from build123d import *

# Parameters (mm, degrees)
F0_R      = 19.7846022737
F1_DEPTH  = 2.794
F1_FACE_R = 19.7846022737
F2_DEPTH  = 6.43804
F2_TAPER  = 45
F2_FACE_R = 13.3465622737
F3_DEPTH  = 12.08628
F3_TAPER  = 3
F4_R      = 10.241679593
F5_DEPTH  = 2.95594
F6_R      = 0.762
F7_R      = 5.08
F8_T      = -2.54
F9_R      = 7.1796509853
F10_DEPTH = 15.93384
F10_TAPER = 3
F11_R     = 4.6826437898
F12_DEPTH = 8.40654


with BuildPart() as f1:
    # F0 (on Top) → F1 (new body)
    with BuildSketch(Plane.XY):
        Circle(F0_R)
    extrude(amount=F1_DEPTH)

    # F1_face (on face) → F2 (join)
    with BuildSketch(Plane.XY.offset(2.794)):
        Circle(F1_FACE_R)
    extrude(amount=F2_DEPTH, taper=F2_TAPER)

    # F2_face (on face) → F3 (join)
    with BuildSketch(Plane.XY.offset(9.23204)):
        Circle(F2_FACE_R)
    extrude(amount=F3_DEPTH, taper=F3_TAPER)

    # F4 (on face) → F5 (cut, symmetric)
    with BuildSketch(Plane.XY.offset(21.31832)):
        Circle(F4_R)
    extrude(amount=F5_DEPTH, both=True, mode=Mode.SUBTRACT)

    # F6
    f6_edges = [f1.edges().sort_by_distance(p)[0] for p in [
        (-12.713147, 0, 21.31832),
        (-10.24168, 0, 21.31832),
    ]]
    fillet(f6_edges, radius=F6_R)

    # F7
    f7_edges = [f1.edges().sort_by_distance(p)[0] for p in [
        (-10.24168, 0, 18.36238),
    ]]
    fillet(f7_edges, radius=F7_R)

    # F8
    f8_openings = [f1.faces().sort_by_distance(p)[0] for p in [
        (0, 0, 0),
    ]]
    offset(amount=F8_T, openings=f8_openings, kind=Kind.INTERSECTION)

    # F9 (on face) → F10 (join)
    with BuildSketch(Plane(origin=(0, 0, 15.82238), x_dir=(1, 0, 0), z_dir=(0, 0, -1))):
        Circle(F9_R)
    extrude(amount=F10_DEPTH, taper=F10_TAPER)

    # F11 (on face) → F12 (cut, symmetric)
    with BuildSketch(Plane(origin=(0, 0, -0.11146), x_dir=(1, 0, 0), z_dir=(0, 0, -1))):
        Circle(F11_R)
    extrude(amount=F12_DEPTH, both=True, mode=Mode.SUBTRACT)


solid = f1.part
Work out the finished part from the listing and answer in its coordinate system (mm). A direction names the side the tool comes from. Coordinates: 2 decimals unless noted, no trailing zeros. Order: outer loops, then holes, each group sorted by start corner. A loop starts at its lowest first (then second) coordinate and runs counter-clockwise, first axis right, second up. Notation, with made-up numbers: (36, 51) - (54, 51) arc R20 cw to (54, 66) - close; hole circle Ø4 at (-26.5, 26.5). An arc over 180 degrees is marked (long way). Put each result on its own line as item: value. Start each with the question number.
1) Flat-ended cylindrical pins translate along their axes: pin 1 (4 mm diameter, centred on x = -4.5, y = 7.5, fed in from +Z); pin 2 (4 mm diameter, centred on y = 14, z = 14.5, fed in from -X); pin 3 (1 mm diameter, centred on x = -6.5, z = 11, fed in from +Y); pin 4 (20.5 mm diameter, centred on x = 0, y = 0, fed in from -Z). Find the tip coordinate at first contact, or state that the pin passes through.
2) Find section B-B (z = 15). Give the vertices of the cut face in (x, y), plus the area to 3 significant figures.
3) Find the intervals of material crossed by line 1 (Y direction, x = 0, z = 1.3); line 2 (Y direction, x = 0, z = 2.5); line 3 (Y direction, x = -4, z = 12.75), in increasing order. Write a range as from..to.
4) Find section A-A (z = 6.5). Give the vertices of the cut face in (x, y).
5) Find section C-C (z = 11.5). Give the vertices of the cut face in (x, y), plus the area to 3 significant figures.
6) For faces 1 (the cylindrical face through (-3.716, 2.849, 4.033)), 2 (the conical face through (-2.961, -13.334, 8.919)), determine the directions among +Z, -Z, +X, -X, +Y, -Y from which every point of the face is accessible in a straight line to the end or side of a thin tool.
7) For a pull along X with two mould halves and no side action, classify faces 3 (the conical face through (5.989, -11.514, 16.256)), 4 (the flat face through (0, 0, 8.295)), 5 (the flat face through (5, -10, 21.318)), 6 (the flat face through (0, 0, 18.362)) as released by +X, released by -X, zero draft, split by the parting line, or undercut.
Results list:
1. pin 1: stops at z = 21.27
1. pin 2: stops at x = -5.19
1. pin 3: stops at y = 11.82
1. pin 4: stops at z = -0.11
2. outline: circle Ø26.09 at (0, 0); circle Ø14.27 at (0, 0); hole circle Ø21 at (0, 0)
2. area: 348 mm^2
3. line 1: y = -19.78..-17.24, -6.42..-4.68, 4.68..6.42, 17.24..19.78
3. line 2: y = -19.78..-16.49, -6.48..-4.68, 4.68..6.48, 16.49..19.78
3. line 3: y = -12.54..-9.84, -5.77..5.77, 9.84..12.54
4. outline: circle Ø32.16 at (0, 0); circle Ø13.38 at (0, 0); hole circle Ø24.97 at (0, 0); hole circle Ø9.37 at (0, 0)
5. outline: circle Ø26.46 at (0, 0); circle Ø13.91 at (0, 0); hole circle Ø21.37 at (0, 0)
5. area: 343 mm^2
6. face 1: -Z
6. face 2: +Z
7. face 3: split by the parting line
7. face 4: undercut
7. face 5: zero draft
7. face 6: undercut
